Solid Edge part; units mm, degrees
sketch "Sketch1" plane through (0, 0, 0) normal (0, 0, 1) x (1, 0, 0)
  circle A0 centre (0, 0) radius 4.25
extrude "Protrusion1" add sketch "Sketch1" along normal blind 5
sketch "Sketch2" plane through (0, 0, 0) normal (0, 0, -1) x (1, 0, 0)
  circle A0 centre (0, 0) radius 2.5
extrude "Protrusion2" add sketch "Sketch2" along normal blind 25
sketch "Sketch3" plane through (0, 0, -25) normal (0, 0, -1) x (1, 0, 0)
  circle A0 centre (0, 0) radius 2.4997
extrude "Cutout1" cut sketch "Sketch3" against normal blind 22 flip side to cut
chamfer "Chamfer_1" distance 0.375 angle 45 1 edges at (-2.4997, 0, -25)
sketch "Sketch4" plane through (0, 0, 5) normal (0, 0, 1) x (1, 0, 0)
  line L0 (-1.1547, 2) -> (1.1547, 2)
  line L1 (2.3094, 0) -> (1.1547, 2)
  line L2 (1.1547, -2) -> (2.3094, 0)
  line L3 (-1.1547, -2) -> (1.1547, -2)
  line L4 (-2.3094, 0) -> (-1.1547, -2)
  line L5 (-1.1547, 2) -> (-2.3094, 0)
extrude "Cutout2" cut sketch "Sketch4" against normal blind 2.5
properties part number "24104801"
Verification items for the finished model (mm, model axes). A direction names the side the tool comes from. Coordinates: 2 decimals unless noted, no trailing zeros. Loops run counter-clockwise (first coordinate to the right, second up) from the corner with the lowest first, then second, coordinate; pieces in that order, holes last. Notation, with made-up numbers: (61, -8.75) -> (72, -8.75) arc R16 ccw to (72, 5.25) -> close; hole circle Ø4 at (25, -33). An arc over 180 degrees is marked (long way). Answer as a JSON object with one key per item and string values. Group by question number.
Item 1: Mould release check, pull along X, two halves, no side actions. Record for faces 4 (the flat face through (0, 2, 4)), 5 (the flat face through (1.724, -1.014, 3.768)), 6 (the cylindrical face through (2.285, -3.584, 2.465)), 7 (the flat face through (2, -1, 5)): +X half, -X half, draft (parallel to the pull), parting line (faces both ways), or undercut.
Item 2: Sectioned sample at D-D on y = -3.25. Record the boundary of the cut face in (x, z).
Item 3: Sectioned sample at B-B on z = -10. Record the boundary of the cut face in (x, y), plus the area to 3 significant figures.
Item 4: Scan lines: probe 1 along Z at (x, y) = (-2.75, -3); probe 2 along Z at (x, y) = (-1, -1.25); probe 3 along Y at (x, z) = (0, 3.25). Record each from-to range of solid material in increasing order.
Item 5: Tool access check on faces 1 (the flat face through (0, 0, -25)), 2 (the cylindrical face through (-2, 1.5, -14)), 3 (the flat face through (0, -2, 4)). Record the directions out of +Z, -Z, +X, -X, +Y, -Y that give a thin tool (end or side, any length) a straight path to the whole face; none if there is none.
Item 6: Depth check by flat-ended pin: pin 1 (2 mm diameter, centred on x = 3, z = -7.5, fed in from +Y); pin 2 (2.5 mm diameter, centred on x = -0.5, z = 4, fed in from -Y); pin 3 (3 mm diameter, centred on x = 0, z = -8.5, fed in from +Y); pin 4 (1.5 mm diameter, centred on y = -3, z = -7.5, fed in from +X). Enter the tip coordinate at first touch or a pass-through.
Item 7: Sectioned sample at C-C on y = 3. Record the boundary of the cut face in (x, z), plus the area to 3 significant figures.
Evaluation:
{
 "1": {"face 4": "undercut", "face 5": "undercut", "face 6": "parting line", "face 7": "draft"},
 "2": {"outline": "(-2.74, 0) -> (2.74, 0) -> (2.74, 5) -> (-2.74, 5) -> close"},
 "3": {"outline": "circle Ø5 at (0, 0)", "area": "19.6 mm²"},
 "4": {"probe 1": "z = 0 to 5", "probe 2": "z = -25 to 2.5", "probe 3": "y = -4.25 to -2, 2 to 4.25"},
 "5": {"face 1": "-Z, +X, -X, +Y, -Y", "face 2": "-Z", "face 3": "+Z"},
 "6": {"pin 1": "stops at y = 1.5", "pin 2": "stops at y = -4.25", "pin 3": "stops at y = 2.5", "pin 4": "stops at x = 1.09"},
 "7": {"outline": "(-3.01, 0) -> (3.01, 0) -> (3.01, 5) -> (-3.01, 5) -> close", "area": "30.1 mm²"}
}
